```python
from build123d import *

# Parameters (mm, degrees)
SKETCH1_R           = 7.85
SKETCH1_R_2         = 1.5
BOSS_EXTRUDE1_DEPTH = 3
SKETCH2_R           = 11.5
SKETCH2_R_2         = 1.5
BOSS_EXTRUDE2_DEPTH = 2
SKETCH3_R           = 3.1
CUT_EXTRUDE1_DEPTH  = 4


with BuildPart() as part:
    # Sketch1 → Boss-Extrude1 (new body)
    with BuildSketch(Plane(origin=(0, 35, 0), x_dir=(1, 0, 0), z_dir=(0, 1, 0))):
        Circle(SKETCH1_R)
        with Locations((-4, 0)):
            Circle(SKETCH1_R_2, mode=Mode.SUBTRACT)
        with Locations((4, 0)):
            Circle(SKETCH1_R_2, mode=Mode.SUBTRACT)
    extrude(amount=BOSS_EXTRUDE1_DEPTH)

    # Sketch2 → Boss-Extrude2 (add)
    with BuildSketch(Plane(origin=(0, 38, 0), x_dir=(1, 0, 0), z_dir=(0, 1, 0))):
        Circle(SKETCH2_R)
        with Locations((-4, 0)):
            Circle(SKETCH2_R_2, mode=Mode.SUBTRACT)
        with Locations((4, 0)):
            Circle(SKETCH2_R_2, mode=Mode.SUBTRACT)
    extrude(amount=BOSS_EXTRUDE2_DEPTH)

    # Sketch3 → Cut-Extrude1 (cut)
    with BuildSketch(Plane(origin=(0, 40, 0), x_dir=(1, 0, 0), z_dir=(0, 1, 0))):
        with Locations((-4, 0)):
            Circle(SKETCH3_R)
        with Locations((4, 0)):
            Circle(SKETCH3_R)
    extrude(amount=-CUT_EXTRUDE1_DEPTH, mode=Mode.SUBTRACT)


solid = part.part
```
Could you check a few things on this model? Use its own coordinates, in mm. A direction names the side the tool comes from. Give positions to 0.01 mm unless a question says otherwise; leave off trailing zeros. Write each loop counter-clockwise with the first axis right and the second up, starting at its lowest first coordinate (ties: lowest second). Pieces come first, ordered by that corner, then holes. Notation, with made-up numbers: (29.25, 69.5) -> (50.25, 69.5) arc R5 cw to (50.25, 74.5) -> close; hole circle Ø1 at (75, 35). An arc over 180 degrees is marked (long way). Write each question's results on one line, items separated by ' | '.
1. If we mould it in two halves opening along X, with no side actions, what happens to faces 1 (the cylindrical face through (1.54, 38.028, 1.886)), 2 (the cylindrical face through (-5.786, 36.479, -5.305)), 3 (the flat face through (0, 40, 0))? For each: released by +X, released by -X, zero draft, split by the parting line, or undercut.
Check sheet entries:
face 1: undercut | face 2: split by the parting line | face 3: zero draft
2. I want a section at C-C, the plane x = 0. Write out the boundary of the cut face in (y, z), then the cut area to 3 significant figures.
Check sheet entries:
outline: (35, -7.85) -> (38, -7.85) -> (38, -11.5) -> (40, -11.5) -> (40, 11.5) -> (38, 11.5) -> (38, 7.85) -> (35, 7.85) -> close | area: 93.1 mm²
3. I want a section at D-D, the plane z = -6.5. Write out the boundary of the cut face in (x, y), then the cut area to 3 significant figures.
Check sheet entries:
outline: (-9.49, 38) -> (-4.4, 38) -> (-4.4, 35) -> (4.4, 35) -> (4.4, 38) -> (9.49, 38) -> (9.49, 40) -> (-9.49, 40) -> close | area: 64.4 mm²
4. On a 3-axis mill with a long thin cutter (end or side, diameter ignored), from which of +Z, -Z, +X, -X, +Y, -Y can I reach the whole of each face in a straight line? I mean faces 4 (the flat face through (8, 38, 2)), 5 (the flat face through (0, 35, 0)), 6 (the cylindrical face through (-7.1, 38, -0.1)). Say none if no direction works.
Check sheet entries:
face 4: -Y | face 5: +Z, -Z, +X, -X, -Y | face 6: +Y
5. I need wall thicknesses on L1, parallel to X at y = 35.4, z = 0; L2, parallel to X at y = 37.05, z = 0; L3, parallel to Y at x = 8, z = -6. Which ranges of each line are inside material? Lowest first, please.
Check sheet entries:
L1: x = -7.85 to -5.5, -2.5 to 2.5, 5.5 to 7.85 | L2: x = -7.85 to -7.1, -0.9 to 0.9, 7.1 to 7.85 | L3: y = 38 to 40
6. Will these pins go through, and if not, where does the flat tip stop? pin 1 Ø2.5 at (x, z) = (-4, 0) entering from +Y; pin 2 Ø7 at (x, z) = (-4, 0) entering from +Y.
Check sheet entries:
pin 1: passes through | pin 2: stops at y = 40
7. I want a section at B-B, the plane x = 4. Write out the boundary of the cut face in (y, z).
Check sheet entries:
outline: (35, -6.75) -> (38, -6.75) -> (38, -10.78) -> (40, -10.78) -> (40, -3.1) -> (36, -3.1) -> (36, -1.5) -> (35, -1.5) -> close; (35, 1.5) -> (36, 1.5) -> (36, 3.1) -> (40, 3.1) -> (40, 10.78) -> (38, 10.78) -> (38, 6.75) -> (35, 6.75) -> close
8. I want a section at A-A, the plane z = 0. Write out the boundary of the cut face in (x, y), then the cut area to 3 significant figures.
Check sheet entries:
outline: (-11.5, 38) -> (-7.85, 38) -> (-7.85, 35) -> (-5.5, 35) -> (-5.5, 36) -> (-7.1, 36) -> (-7.1, 40) -> (-11.5, 40) -> close; (-2.5, 35) -> (2.5, 35) -> (2.5, 36) -> (0.9, 36) -> (0.9, 40) -> (-0.9, 40) -> (-0.9, 36) -> (-2.5, 36) -> close; (5.5, 35) -> (7.85, 35) -> (7.85, 38) -> (11.5, 38) -> (11.5, 40) -> (7.1, 40) -> (7.1, 36) -> (5.5, 36) -> close | area: 37.5 mm²
